```python
from build123d import *

# Parameters (mm, degrees)
DODANIE_WYCI_GNI_CIE1_DEPTH = 1260
SZKIC6_R                    = 6.5
WYTNIJ_WYCI_GNI_CIE5_DEPTH  = 30


with BuildPart() as part:
    # Szkic1 → Dodanie-wyciągnięcie1 (new body)
    with BuildSketch(Plane.XY):
        with BuildLine():
            Line((-12, -15), (12, -15))
            ThreePointArc((12, -15), (14.121320344, -14.121320344), (15, -12))
            Line((15, -12), (15, 12))
            ThreePointArc((15, 12), (14.121320344, 14.121320344), (12, 15))
            Line((12, 15), (-12, 15))
            ThreePointArc((-12, 15), (-14.121320344, 14.121320344), (-15, 12))
            Line((-15, 12), (-15, -12))
            ThreePointArc((-15, -12), (-14.121320344, -14.121320344), (-12, -15))
        make_face()
        with BuildLine():
            Line((-11, -12), (11, -12))
            ThreePointArc((11, -12), (11.707106781, -11.707106781), (12, -11))
            Line((12, -11), (12, 11))
            ThreePointArc((12, 11), (11.707106781, 11.707106781), (11, 12))
            Line((11, 12), (-11, 12))
            ThreePointArc((-11, 12), (-11.707106781, 11.707106781), (-12, 11))
            Line((-12, 11), (-12, -11))
            ThreePointArc((-12, -11), (-11.707106781, -11.707106781), (-11, -12))
        make_face(mode=Mode.SUBTRACT)
    extrude(amount=DODANIE_WYCI_GNI_CIE1_DEPTH)

    # Szkic6 → Wytnij-wyciągnięcie5 (cut)
    with BuildSketch(Plane(origin=(0, 15, 0), x_dir=(1, 0, 0), z_dir=(0, 1, 0))):
        with Locations((0, -948.6)):
            Circle(SZKIC6_R)
        with Locations((0, -698.6)):
            Circle(SZKIC6_R)
    extrude(amount=-WYTNIJ_WYCI_GNI_CIE5_DEPTH, mode=Mode.SUBTRACT)


solid = part.part
```
Can you work these out from the model? Positions are in its coordinate system, mm. A direction names the side the tool comes from. Coordinates: 2 decimals unless noted, no trailing zeros. Loops run counter-clockwise (first coordinate to the right, second up) from the corner with the lowest first, then second, coordinate; pieces in that order, holes last. Notation, with made-up numbers: (-7.5, 61.25) - (46.5, 61.25) arc R23 ccw to (46.5, 87.25) - close; hole circle Ø4 at (-19.75, 69). An arc over 180 degrees is marked (long way). Use a Markdown table: item, result.
Item 1: I want a section at B-B on z = 924. Please give me the cut outline in (x, y), and give its area (3 significant figures).
Numbers:
| item | result |
|---|---|
| outline | (-15, -12) arc R3 ccw to (-12, -15) - (12, -15) arc R3 ccw to (15, -12) - (15, 12) arc R3 ccw to (12, 15) - (-12, 15) arc R3 ccw to (-15, 12) - close; hole (-12, -11) arc R1 ccw to (-11, -12) - (11, -12) arc R1 ccw to (12, -11) - (12, 11) arc R1 ccw to (11, 12) - (-11, 12) arc R1 ccw to (-12, 11) - close |
| area | 317 mm2 |
Item 2: For faces 4 (the face through (12, 0, 621)), 5 (the face through (-14, 0, 0)), which set-ups out of +Z, -Z, +X, -X, +Y, -Y let a thin tool reach every point of the face, with its end or its side?
Numbers:
| item | result |
|---|---|
| face 4 | +Z, -Z |
| face 5 | -Z, +X, -X, +Y, -Y |
Item 3: If I drill on probe 1 along Z at (x, y) = (0, -12.95); probe 2 along Y at (x, z) = (-5, 373), over which ranges is the centre line in solid material (lowest first)? Write a range as from..to.
Numbers:
| item | result |
|---|---|
| probe 1 | z = 0..692.1, 705.1..942.1, 955.1..1260 |
| probe 2 | y = -15..-12, 12..15 |
Item 4: I want a section at A-A on y = -0.25. Please give me the cut outline in (x, z).
Numbers:
| item | result |
|---|---|
| outline | (-15, 0) - (-12, 0) - (-12, 1260) - (-15, 1260) - close; (12, 0) - (15, 0) - (15, 1260) - (12, 1260) - close |
Item 5: We'd pull the mould along Y, two halves only. Please class faces 1 (the face through (0, -12, 621)), 2 (the face through (0, 15, 621)), 3 (the face through (-14, 0, 1260)): released by +Y, released by -Y, zero draft, split by the parting line, or undercut.
Numbers:
| item | result |
|---|---|
| face 1 | undercut |
| face 2 | released by +Y |
| face 3 | zero draft |
Item 6: I want a section at C-C on x = 0. Please give me the cut outline in (y, z), and give its area (3 significant figures).
Numbers:
| item | result |
|---|---|
| outline | (-15, 0) - (-12, 0) - (-12, 692.1) - (-15, 692.1) - close; (-15, 705.1) - (-12, 705.1) - (-12, 942.1) - (-15, 942.1) - close; (-15, 955.1) - (-12, 955.1) - (-12, 1260) - (-15, 1260) - close; (12, 0) - (15, 0) - (15, 692.1) - (12, 692.1) - close; (12, 705.1) - (15, 705.1) - (15, 942.1) - (12, 942.1) - close; (12, 955.1) - (15, 955.1) - (15, 1260) - (12, 1260) - close |
| area | 7,400 mm2 |
Item 7: Will this pin go through, and if not, where does the flat tip stop? pin 1 (8 mm diameter, centred on x = -2, y = 4.5, fed in from -Z).
Numbers:
| item | result |
|---|---|
| pin 1 | passes through |
